Here's how the part is built. I have some questions about the finished solid (model axes, mm). Give positions to 0.01 mm unless a question says otherwise; leave off trailing zeros. Write each loop counter-clockwise with the first axis right and the second up, starting at its lowest first coordinate (ties: lowest second). Pieces come first, ordered by that corner, then holes. Notation, with made-up numbers: (52.25, -5.75) - (92.25, -5.75) arc R27 cw to (92.25, 26.25) - close; hole circle Ø2 at (-5, 88.5). An arc over 180 degrees is marked (long way). Write each question's results on one line, items separated by ' | '. Start each with the question number.
Item 1: Suppose I cut it at A-A on z = 50. List the corners of the cut face in (x, y) for me, then the cut area to 3 significant figures.
Item 2: Will these pins go through, and if not, where does the flat tip stop? P1, Ø16, axis at x = 50, z = -50, coming from the +Y side; P2, Ø3, axis at x = -15.5, y = -3.5, coming from the +Z side; P3, Ø5, axis at x = -21, y = -5.5, coming from the -Z side; P4, Ø5, axis at y = -6, z = 24.5, coming from the +X side.
Item 3: Suppose I cut it at C-C on x = -50. List the corners of the cut face in (y, z) for me, then the cut area to 3 significant figures.
Item 4: Please list where these lines run through material, in increasing order: line 1 along Z through (x, y) = (-50, -4); line 2 along X through (y, z) = (2.5, -50); line 3 along Z through (x, y) = (49, -5.25).
Item 5: Suppose I cut it at B-B on y = -7.5. List the corners of the cut face in (x, z) for me.
Item 6: Suppose I cut it at D-D on y = 6.5. Count the separate pieces of the cut face and the enclosed holes in it, then the cut area to 3 significant figures.
```python
from build123d import *

# Parameters (mm, degrees)
CROQUIS1_W              = 200
CROQUIS1_H              = 200
SALIENTE_EXTRUIR1_DEPTH = 10
CROQUIS2_W              = 194
CROQUIS2_H              = 187
SALIENTE_EXTRUIR2_DEPTH = 10
REDONDEO2_R             = 4.5
CROQUIS3_R              = 10
CORTAR_EXTRUIR1_DEPTH   = 20
CROQUIS4_R              = 1.6
CORTAR_EXTRUIR2_DEPTH   = 10


with BuildPart() as part:
    # Croquis1 → Saliente-Extruir1 (new body)
    with BuildSketch(Plane(origin=(0, 0, 0), x_dir=(1, 0, 0), z_dir=(0, 1, 0))):
        Rectangle(CROQUIS1_W, CROQUIS1_H)
    extrude(amount=SALIENTE_EXTRUIR1_DEPTH)

    # Croquis2 → Saliente-Extruir2 (add)
    with BuildSketch(Plane.XZ):
        with Locations((0, 3.5)):
            Rectangle(CROQUIS2_W, CROQUIS2_H)
    extrude(amount=SALIENTE_EXTRUIR2_DEPTH)

    # Redondeo2
    redondeo2_edges = [part.edges().sort_by_distance(p)[0] for p in [
        (-97, -5, 97),
        (-97, -5, -90),
        (97, -5, -90),
        (97, -5, 97),
    ]]
    fillet(redondeo2_edges, radius=REDONDEO2_R)

    # Croquis3 → Cortar-Extruir1 (cut)
    with BuildSketch(Plane(origin=(0, 10, 0), x_dir=(1, 0, 0), z_dir=(0, 1, 0))):
        with Locations((-50, 50)):
            Circle(CROQUIS3_R)
        with Locations((-50, 0)):
            Circle(CROQUIS3_R)
        with Locations((-50, -50)):
            Circle(CROQUIS3_R)
    cortar_extruir1 = extrude(amount=-CORTAR_EXTRUIR1_DEPTH, mode=Mode.SUBTRACT)

    # Simetría1: Cortar-Extruir1 across plane
    add(cortar_extruir1.mirror(Plane(origin=(0, 0, 0), x_dir=(0, 0, 1), z_dir=(1, 0, 0))), mode=Mode.SUBTRACT)

    # Croquis4 → Cortar-Extruir2 (cut)
    with BuildSketch(Plane(origin=(0, 10, 0), x_dir=(1, 0, 0), z_dir=(0, 1, 0))):
        with Locations((-70, 95)):
            Circle(CROQUIS4_R)
        with Locations((-41, 95)):
            Circle(CROQUIS4_R)
    cortar_extruir2 = extrude(amount=-CORTAR_EXTRUIR2_DEPTH, mode=Mode.SUBTRACT)

    # Simetría2: Cortar-Extruir2 across plane
    add(cortar_extruir2.mirror(Plane(origin=(0, 0, 0), x_dir=(0, 0, 1), z_dir=(1, 0, 0))), mode=Mode.SUBTRACT)


solid = part.part
```
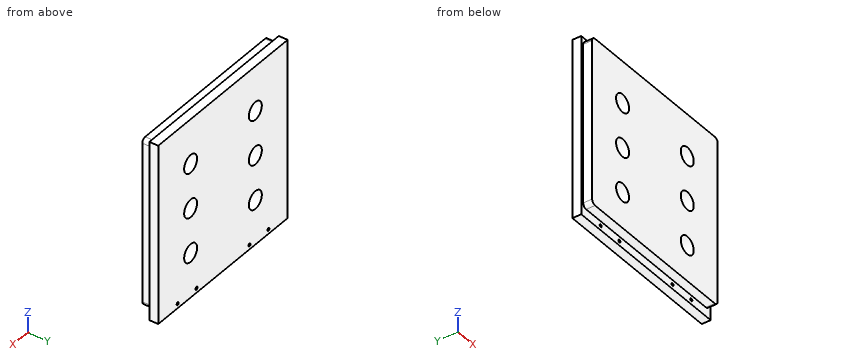
Checked values:
1) outline: (-100, 0) - (-97, 0) - (-97, -10) - (-60, -10) - (-60, 10) - (-100, 10) - close; (-40, -10) - (40, -10) - (40, 10) - (-40, 10) - close; (60, -10) - (97, -10) - (97, 0) - (100, 0) - (100, 10) - (60, 10) - close | area: 3,140 mm^2
2) P1: passes through | P2: stops at z = 97 | P3: stops at z = -90 | P4: stops at x = 97
3) outline: (-10, -90) - (0, -90) - (0, -100) - (10, -100) - (10, -60) - (-10, -60) - close; (-10, -40) - (10, -40) - (10, -10) - (-10, -10) - close; (-10, 10) - (10, 10) - (10, 40) - (-10, 40) - close; (-10, 60) - (10, 60) - (10, 100) - (0, 100) - (0, 97) - (-10, 97) - close | area: 2,670 mm^2
4) line 1: z = -90 to -60, -40 to -10, 10 to 40, 60 to 97 | line 2: x = -100 to -60, -40 to 40, 60 to 100 | line 3: z = -90 to -59.95, -40.05 to -9.95, 9.95 to 40.05, 59.95 to 97
5) outline: (-97, -85.5) arc R4.5 ccw to (-92.5, -90) - (92.5, -90) arc R4.5 ccw to (97, -85.5) - (97, 92.5) arc R4.5 ccw to (92.5, 97) - (-92.5, 97) arc R4.5 ccw to (-97, 92.5) - close; hole circle Ø20 at (-50, -50); hole circle Ø20 at (-50, 0); hole circle Ø20 at (-50, 50); hole circle Ø20 at (50, -50); hole circle Ø20 at (50, 0); hole circle Ø20 at (50, 50)
6) separate pieces: 1 | enclosed holes: 10 | area: 38,100 mm^2
